The listing builds one solid part. Answer for the finished solid, in the listing's coordinates (mm). A direction names the side the tool comes from. Round coordinates to 2 decimals unless told otherwise and drop trailing zeros. Write each loop counter-clockwise with the first axis right and the second up, starting at its lowest first coordinate (ties: lowest second). Pieces come first, ordered by that corner, then holes.
Item 1: A tool of negligible diameter and unlimited length cuts with its end or side. For faces 1 (the face through (-277.276, 151, 163)), 2 (the face through (-787.4, 150, 150)), from which of +Z, -Z, +X, -X, +Y, -Y can it reach the whole face along a straight path? Write none if from no direction.
Item 2: Find the intervals of material crossed by probe 1 along X at (y, z) = (189, 216.5); probe 2 along Y at (x, z) = (-332.5, 54.5); probe 3 along Z at (x, y) = (-77, 56.5), in increasing order.
Item 3: For a pull along Y with two mould halves and no side action, classify faces 3 (the face through (-759.876, 151, 167)), 4 (the face through (-399, 0, 150)), 5 (the face through (-23.276, 151, 167)), 6 (the face through (0, 150, 150)) as +Y half, -Y half, draft (parallel to the pull), parting line (faces both ways), or undercut.
Item 4: Find section C-C on x = -708.5. Give the vertices of the cut face in (y, z).
Item 5: Find section A-A on y = 194.5. Give the vertices of the cut face in (x, z), then the cut area to 3 significant figures.
Item 6: Find section B-B on z = 203. Give the vertices of the cut face in (x, y).
```python
from build123d import *

# Parameters (mm, degrees)
F0_W     = 787.4
F0_H     = 304.8
F1_DEPTH = 304.8
F2_W     = 228.6
F2_H     = 254
F2_W_2   = 508
F4_DEPTH = 279.4
F3_W     = 508
F3_H     = 254
F5_DEPTH = 279.4
F6_W     = 25.4
F6_H     = 254
F7_DEPTH = 279.4
F8_W     = 25.4
F8_H     = 254
F9_DEPTH = 279.4


with BuildPart() as f1:
    # F0 (on Top) → F1 (new body)
    with BuildSketch(Plane.XY):
        with Locations((-393.7, 152.4)):
            Rectangle(F0_W, F0_H)
    extrude(amount=F1_DEPTH)

    # F2 (on face) → F4 (cut)
    with BuildSketch(Plane.XY.offset(304.8)):
        with Locations((-645.575834, 152.4)):
            Rectangle(F2_W, F2_H)
        with Locations((-277.275834, 152.4)):
            Rectangle(F2_W_2, F2_H)
    extrude(amount=-F4_DEPTH, mode=Mode.SUBTRACT)

    # F3 (on face) → F5 (cut)
    with BuildSketch(Plane.XY.offset(304.8)):
        with Locations((-277.275834, 152.4)):
            Rectangle(F3_W, F3_H)
    extrude(amount=-F5_DEPTH, mode=Mode.SUBTRACT)

    # F6 (on face) → F7 (join, through all)
    with BuildSketch(Plane.XY.offset(25.4)):
        with Locations((-518.575834, 152.4)):
            Rectangle(F6_W, F6_H)
    extrude(amount=F7_DEPTH)

    # F8 (on face) → F9 (join, through all)
    with BuildSketch(Plane.XY.offset(25.4)):
        with Locations((-264.575834, 152.4)):
            Rectangle(F8_W, F8_H)
    extrude(amount=F9_DEPTH)


solid = f1.part
```
Check values:
1. face 1: +Z
1. face 2: +Z, -Z, -X, +Y, -Y
2. probe 1: x = -787.4 to -759.88, -531.28 to -505.88, -277.28 to -251.88, -23.28 to 0
2. probe 2: y = 0 to 25.4, 279.4 to 304.8
2. probe 3: z = 0 to 25.4
3. face 3: undercut
3. face 4: -Y half
3. face 5: undercut
3. face 6: draft
4. outline: (0, 0) - (304.8, 0) - (304.8, 304.8) - (279.4, 304.8) - (279.4, 25.4) - (25.4, 25.4) - (25.4, 304.8) - (0, 304.8) - close
5. outline: (-787.4, 0) - (0, 0) - (0, 304.8) - (-23.28, 304.8) - (-23.28, 25.4) - (-251.88, 25.4) - (-251.88, 304.8) - (-277.28, 304.8) - (-277.28, 25.4) - (-505.88, 25.4) - (-505.88, 304.8) - (-531.28, 304.8) - (-531.28, 25.4) - (-759.88, 25.4) - (-759.88, 304.8) - (-787.4, 304.8) - close
5. area: 48,400 mm2
6. outline: (-787.4, 0) - (0, 0) - (0, 304.8) - (-787.4, 304.8) - close; hole (-759.88, 25.4) - (-531.28, 25.4) - (-531.28, 279.4) - (-759.88, 279.4) - close; hole (-505.88, 25.4) - (-277.28, 25.4) - (-277.28, 279.4) - (-505.88, 279.4) - close; hole (-251.88, 25.4) - (-23.28, 25.4) - (-23.28, 279.4) - (-251.88, 279.4) - close
